from build123d import *

# Parameters (mm, degrees)
SKETCH1_R           = 2.6
BOSS_EXTRUDE1_DEPTH = 3
SKETCH2_W           = 3
SKETCH2_H           = 3.2
SKETCH2_W_2         = 19
SKETCH2_R           = 1.6
CUT_EXTRUDE1_DEPTH  = 10
FILLET1_R           = 5
SKETCH3_R           = 1.6
CUT_EXTRUDE2_DEPTH  = 321.989096388


with BuildPart() as part:
    # Sketch1 → Boss-Extrude1 (new body)
    # profile 1 of 2: a face of its own
    with BuildSketch(Plane(origin=(0, 0, 0), x_dir=(1, 0, 0), z_dir=(0, 1, 0))):
        with BuildLine():
            Line((0, -45), (260, -45))
            ThreePointArc((260, -45), (305, 0), (260, 45))
            Line((260, 45), (0, 45))
            ThreePointArc((0, 45), (-45, 0), (0, -45))
        make_face()
        with Locations(Location((0, 0, 0), (0, 0, 270))):
            Circle(SKETCH1_R, mode=Mode.SUBTRACT)
        with BuildLine():
            ThreePointArc((250, 2.6), (247.4, 0), (250, -2.6))
            Line((250, -2.6), (270, -2.6))
            ThreePointArc((270, -2.6), (272.6, 0), (270, 2.6))
            Line((270, 2.6), (250, 2.6))
        make_face(mode=Mode.SUBTRACT)
    # profile 2 of 2: a face of its own
    with BuildSketch(Plane(origin=(0, 0, 0), x_dir=(1, 0, 0), z_dir=(0, 1, 0))):
        with BuildLine():
            ThreePointArc((-45, 0), (-31.819805153, 31.819805153), (0, 45))
            Line((0, 45), (260, 45))
            ThreePointArc((260, 45), (291.819805153, 31.819805153), (305, 0))
            Line((305, 0), (305, 100))
            Line((305, 100), (-45, 100))
            Line((-45, 100), (-45, 0))
        make_face()
    extrude(amount=BOSS_EXTRUDE1_DEPTH)

    # Sketch2 → Cut-Extrude1 (cut)
    with BuildSketch(Plane.XZ):
        with Locations((81.5, -35)):
            Rectangle(SKETCH2_W, SKETCH2_H)
        with BuildLine():
            Line((80, -33.4), (83, -33.4))
            ThreePointArc((83, -33.4), (81.5, -31.9), (80, -33.4))
        make_face()
        with BuildLine():
            ThreePointArc((80, -36.6), (81.5, -38.1), (83, -36.6))
            Line((83, -36.6), (80, -36.6))
        make_face()
        with Locations((92.5, -35)):
            Rectangle(SKETCH2_W_2, SKETCH2_H)
        with BuildLine():
            ThreePointArc((105, -33.4), (103.5, -31.9), (102, -33.4))
            Line((102, -33.4), (105, -33.4))
        make_face()
        with Locations((103.5, -35)):
            Rectangle(SKETCH2_W, SKETCH2_H)
        with BuildLine():
            Line((105, -36.6), (102, -36.6))
            ThreePointArc((102, -36.6), (103.5, -38.1), (105, -36.6))
        make_face()
        with BuildLine():
            ThreePointArc((83, -73.4), (81.5, -71.9), (80, -73.4))
            Line((80, -73.4), (83, -73.4))
        make_face()
        with Locations((81.5, -75)):
            Rectangle(SKETCH2_W, SKETCH2_H)
        with Locations((92.5, -75)):
            Rectangle(SKETCH2_W_2, SKETCH2_H)
        with BuildLine():
            Line((83, -76.6), (80, -76.6))
            ThreePointArc((80, -76.6), (81.5, -78.1), (83, -76.6))
        make_face()
        with BuildLine():
            ThreePointArc((105, -73.4), (103.5, -71.9), (102, -73.4))
            Line((102, -73.4), (105, -73.4))
        make_face()
        with Locations((103.5, -75)):
            Rectangle(SKETCH2_W, SKETCH2_H)
        with BuildLine():
            Line((105, -76.6), (102, -76.6))
            ThreePointArc((102, -76.6), (103.5, -78.1), (105, -76.6))
        make_face()
        with BuildLine():
            Line((155, -33.4), (158, -33.4))
            ThreePointArc((158, -33.4), (156.5, -31.9), (155, -33.4))
        make_face()
        with Locations((156.5, -35)):
            Rectangle(SKETCH2_W, SKETCH2_H)
        with BuildLine():
            ThreePointArc((155, -36.6), (156.5, -38.1), (158, -36.6))
            Line((158, -36.6), (155, -36.6))
        make_face()
        with Locations((167.5, -35)):
            Rectangle(SKETCH2_W_2, SKETCH2_H)
        with BuildLine():
            Line((177, -33.4), (180, -33.4))
            ThreePointArc((180, -33.4), (178.5, -31.9), (177, -33.4))
        make_face()
        with Locations((178.5, -35)):
            Rectangle(SKETCH2_W, SKETCH2_H)
        with BuildLine():
            ThreePointArc((177, -36.6), (178.5, -38.1), (180, -36.6))
            Line((180, -36.6), (177, -36.6))
        make_face()
        with BuildLine():
            ThreePointArc((158, -73.4), (156.5, -71.9), (155, -73.4))
            Line((155, -73.4), (158, -73.4))
        make_face()
        with Locations((156.5, -75)):
            Rectangle(SKETCH2_W, SKETCH2_H)
        with BuildLine():
            Line((158, -76.6), (155, -76.6))
            ThreePointArc((155, -76.6), (156.5, -78.1), (158, -76.6))
        make_face()
        with Locations((167.5, -75)):
            Rectangle(SKETCH2_W_2, SKETCH2_H)
        with BuildLine():
            ThreePointArc((180, -73.4), (178.5, -71.9), (177, -73.4))
            Line((177, -73.4), (180, -73.4))
        make_face()
        with Locations((178.5, -75)):
            Rectangle(SKETCH2_W, SKETCH2_H)
        with BuildLine():
            Line((180, -76.6), (177, -76.6))
            ThreePointArc((177, -76.6), (178.5, -78.1), (180, -76.6))
        make_face()
        with Locations(Location((200, -75, 0), (0, 0, 270))):
            Circle(SKETCH2_R)
        with Locations(Location((290, -92, 0), (0, 0, 270))):
            Circle(SKETCH2_R)
        with Locations(Location((270, -92, 0), (0, 0, 270))):
            Circle(SKETCH2_R)
        with Locations(Location((60, -35, 0), (0, 0, 90))):
            Circle(SKETCH2_R)
        with Locations(Location((60, -75, 0), (0, 0, 270))):
            Circle(SKETCH2_R)
        with Locations(Location((-10, -92, 0), (0, 0, 270))):
            Circle(SKETCH2_R)
        with Locations(Location((-30, -92, 0), (0, 0, 270))):
            Circle(SKETCH2_R)
        with Locations(Location((200, -35, 0), (0, 0, 270))):
            Circle(SKETCH2_R)
    extrude(amount=-CUT_EXTRUDE1_DEPTH, mode=Mode.SUBTRACT)

    # Fillet1
    fillet1_edges = [part.edges().sort_by_distance(p)[0] for p in [
        (-45, 1.5, -100),
        (305, 1.5, -100),
    ]]
    fillet(fillet1_edges, radius=FILLET1_R)

    # Sketch3 → Cut-Extrude2 (cut, through all)
    with BuildSketch(Plane.XZ):
        with Locations(Location((105, 35, 0), (0, 0, 270))):
            Circle(SKETCH3_R)
        with Locations(Location((155, 35, 0), (0, 0, 270))):
            Circle(SKETCH3_R)
        with BuildLine():
            Line((193.4, -1.6), (153.4, -1.6))
            ThreePointArc((153.4, -1.6), (151.8, 0), (153.4, 1.6))
            Line((153.4, 1.6), (193.4, 1.6))
            ThreePointArc((193.4, 1.6), (195, 0), (193.4, -1.6))
        make_face()
    extrude(amount=-CUT_EXTRUDE2_DEPTH, mode=Mode.SUBTRACT)


solid = part.part
Here's how the part is built. I have some questions about the finished solid (model axes, mm). Round coordinates to 2 decimals unless told otherwise and drop trailing zeros. Loops run counter-clockwise (first coordinate to the right, second up) from the corner with the lowest first, then second, coordinate; pieces in that order, holes last. Notation, with made-up numbers: M 8.5,-6 L 14.5,-6 A19 ccw 14.5,24 Z; hole C 31.25,78.5 d5. An arc over 180 degrees is marked long. Write each question's results on one line, items separated by ' | '. Start each with the question number.
(1) Will this pin go through, and if not, where does the flat tip stop? P1, Ø1, axis at y = 0.5, z = 19.5, coming from the +X side.
(2) I want a section at A-A (y = 1.2). State how many separate pieces and enclosed holes the cut face has, then the cut area to 3 significant figures.
(3) If I drill on probe 1 along X at (y, z) = (1.95, 0); probe 2 along X at (y, z) = (1.45, -35); probe 3 along Z at (x, y) = (164, 2.6), over which ranges is the centre line in solid material (lowest first)? Write a range as from..to.
(4) I want a section at B-B (z = 25). Please give me the cut outline in (x, y), then the cut area to 3 significant figures.
Solved:
1) P1: stops at x = 300.79
2) separate pieces: 1 | enclosed holes: 17 | area: 49,100 mm²
3) probe 1: x = -45..-2.6, 2.6..151.8, 195..247.4, 272.6..305 | probe 2: x = -45..58.4, 61.6..80, 105..155, 180..198.4, 201.6..305 | probe 3: z = -100..-76.6, -73.4..-36.6, -33.4..-1.6, 1.6..45
4) outline: M -37.42,0 L 297.42,0 L 297.42,3 L -37.42,3 Z | area: 1,000 mm²
